Geometry: see drawing. Coordinates: mm, zero at the bounding-box minimum. A direction names the side the tool comes from. Round coordinates to 2 decimals unless told otherwise and drop trailing zeros. Loops run counter-clockwise (first coordinate to the right, second up) from the corner with the lowest first, then second, coordinate; pieces in that order, holes last. Notation, with made-up numbers: (36, 57.5) - (84, 57.5) arc R16 ccw to (84, 61.5) - close; hole circle Ø1 at (-36.5, -6.5). An arc over 180 degrees is marked (long way). Use CSV: the item, a comma, the result in double quotes.
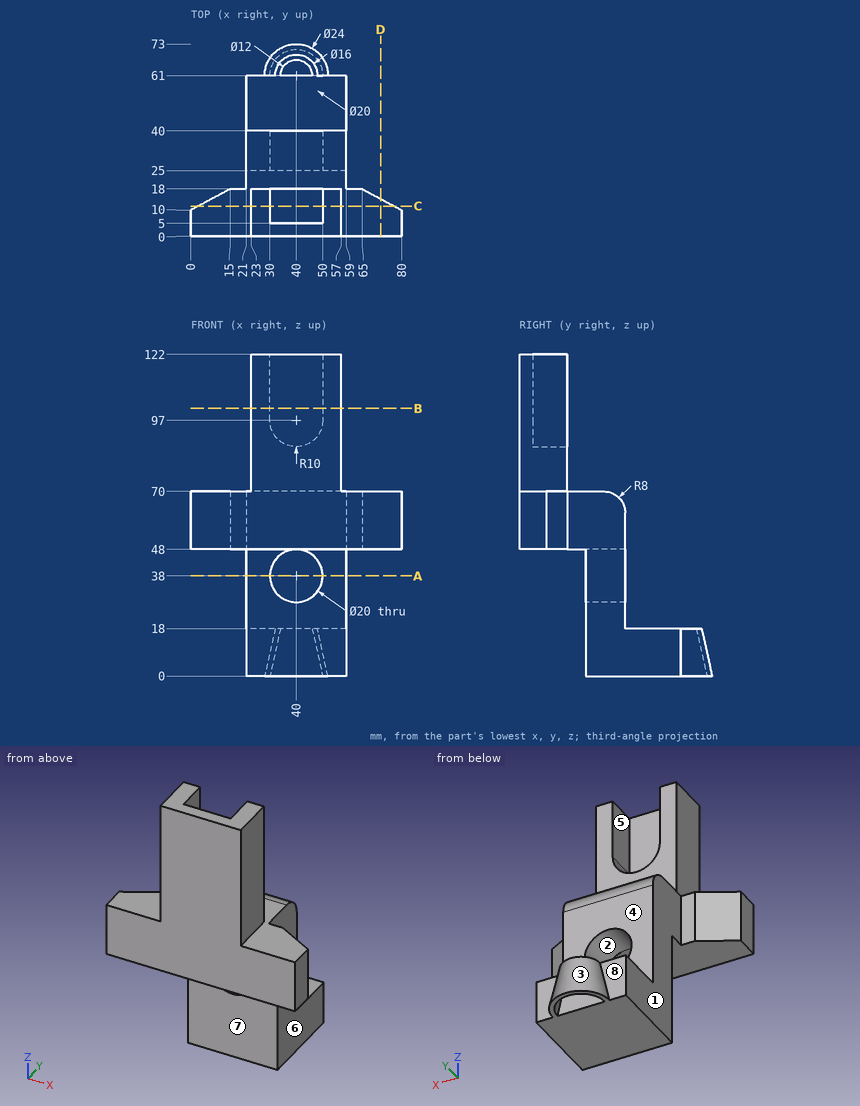
Item 1: Reachability of the marked faces 4, 5, 6, 7 and 8 from +Z, -Z, +X, -X, +Y, -Y: full face, straight path, thin tool, end or side. Return the list, or none.
Final values:
face 4,"+Z, +X, -X, +Y"
face 5,"+Z, +Y"
face 6,"+Z, -Z, +X, +Y"
face 7,"-Z, +X, -X, -Y"
face 8,"+Z, -X, +Y"
Item 2: Section A-A on z = 38. Return the cut outline in (x, y).
Final values:
outline,"(21, 25) - (30, 25) - (30, 40) - (21, 40) - close; (50, 25) - (59, 25) - (59, 40) - (50, 40) - close"
Item 3: Section C-C on y = 11.5. Return the cut outline in (x, z).
Final values:
outline,"(2.81, 48) - (77.19, 48) - (77.19, 70) - (57, 70) - (57, 122) - (50, 122) - (50, 97) arc R10 cw to (30, 97) - (30, 122) - (23, 122) - (23, 70) - (2.81, 70) - close"
Item 4: Section B-B on z = 101.5. Return the cut outline in (x, y), plus the area to 3 significant figures.
Final values:
outline,"(23, 0) - (57, 0) - (57, 18) - (50, 18) - (50, 5) - (30, 5) - (30, 18) - (23, 18) - close"
area,"352 mm²"
Item 5: Mould query, pull axis X, two halves, no side actions, for the marked faces 1, 2 and 3. Classes: released by +X, released by -X, zero draft, split by the parting line, or undercut.
Final values:
face 1,"released by -X"
face 2,"undercut"
face 3,"split by the parting line"
Item 6: Pin query (flat end, axial travel): P1, Ø4, axis at x = 54.5, y = 57, coming from the +Z side; P2, Ø16, axis at x = 42.5, z = 111, coming from the +Y side; P3, Ø20, axis at x = 40, y = 10.5, coming from the -Z side. Return the tip coordinate at first contact, or that it passes through.
Final values:
P1,"stops at z = 18"
P2,"stops at y = 18"
P3,"stops at z = 48"
Item 7: Section D-D on x = 72. Return the cut outline in (y, z), plus the area to 3 significant figures.
Final values:
outline,"(0, 48) - (14.27, 48) - (14.27, 70) - (0, 70) - close"
area,"314 mm²"
Item 8: Material intervals for line 1 (X direction, y = 36.5, z = 38); line 2 (Z direction, x = 40, y = 28); line 3 (Y direction, x = 38.5, z = 86), sorted ascending.
Final values:
line 1,"x = 21 to 30, 50 to 59"
line 2,"z = 0 to 28, 48 to 70"
line 3,"y = 0 to 18"
